```python
from build123d import *

# Parameters (mm, degrees)
SKIZZE1_W                       = 20
SKIZZE1_H                       = 10
AUFSATZ_LINEAR_AUSTRAGEN1_DEPTH = 10
SKIZZE3_W                       = 4.1
SKIZZE3_H                       = 1.9
SCHNITT_LINEAR_AUSTRAGEN2_DEPTH = 5
SKIZZE9_RX                      = 9
SKIZZE9_RY                      = 3
SCHNITT_LINEAR_AUSTRAGEN3_DEPTH = 10
SKIZZE10_W                      = 6.95
SKIZZE10_H                      = 5
SCHNITT_LINEAR_AUSTRAGEN4_DEPTH = 1.5
SKIZZE11_W                      = 7
SKIZZE11_H                      = 5
SCHNITT_LINEAR_AUSTRAGEN5_DEPTH = 1.5
SKIZZE13_W                      = 1
SKIZZE13_H                      = 1
SCHNITT_LINEAR_AUSTRAGEN7_DEPTH = 10
SKIZZE14_W                      = 0.5
SKIZZE14_H                      = 0.5
SCHNITT_LINEAR_AUSTRAGEN8_DEPTH = 10
VERRUNDUNG2_R                   = 0.2
VERRUNDUNG3_R                   = 0.2
VERRUNDUNG4_R                   = 0.2
VERRUNDUNG5_R                   = 0.2
VERRUNDUNG6_R                   = 0.2


with BuildPart() as part:
    # Skizze1 → Aufsatz-Linear austragen1 (new body)
    with BuildSketch(Plane.XY):
        with Locations((-10, 2.346944746)):
            Rectangle(SKIZZE1_W, SKIZZE1_H)
    extrude(amount=AUFSATZ_LINEAR_AUSTRAGEN1_DEPTH)

    # Skizze3 → Schnitt-Linear austragen2 (cut)
    with BuildSketch(Plane(origin=(0, 0, 0), x_dir=(-1, 0, 0), z_dir=(0, 0, -1))):
        with Locations((10, 2.346944746)):
            Rectangle(SKIZZE3_W, SKIZZE3_H)
    extrude(amount=-SCHNITT_LINEAR_AUSTRAGEN2_DEPTH, mode=Mode.SUBTRACT)

    # Skizze9 → Schnitt-Linear austragen3 (cut)
    with BuildSketch(Plane(origin=(0, 7.346944746, 0), x_dir=(1, 0, 0), z_dir=(0, 1, 0))):
        with Locations((-10, -10)):
            Ellipse(SKIZZE9_RX, SKIZZE9_RY)
    extrude(amount=-SCHNITT_LINEAR_AUSTRAGEN3_DEPTH, mode=Mode.SUBTRACT)

    # Skizze10 → Schnitt-Linear austragen4 (cut)
    with BuildSketch(Plane(origin=(0, 0, 0), x_dir=(-1, 0, 0), z_dir=(0, 0, -1))):
        with Locations((16.525, 2.021356222)):
            Rectangle(SKIZZE10_W, SKIZZE10_H)
    extrude(amount=-SCHNITT_LINEAR_AUSTRAGEN4_DEPTH, mode=Mode.SUBTRACT)

    # Skizze11 → Schnitt-Linear austragen5 (cut)
    with BuildSketch(Plane(origin=(0, 0, 0), x_dir=(-1, 0, 0), z_dir=(0, 0, -1))):
        with Locations((3.5, 2.346944746)):
            Rectangle(SKIZZE11_W, SKIZZE11_H)
    extrude(amount=-SCHNITT_LINEAR_AUSTRAGEN5_DEPTH, mode=Mode.SUBTRACT)

    # Skizze13 → Schnitt-Linear austragen7 (cut)
    with BuildSketch(Plane.XZ.offset(2.653055254)):
        with Locations((-10, 6.665824705)):
            Rectangle(SKIZZE13_W, SKIZZE13_H)
    extrude(amount=-SCHNITT_LINEAR_AUSTRAGEN7_DEPTH, mode=Mode.SUBTRACT)

    # Skizze14 → Schnitt-Linear austragen8 (cut)
    with BuildSketch(Plane.XZ.offset(2.653055254)):
        with Locations((-15.25, 7.45)):
            Rectangle(SKIZZE14_W, SKIZZE14_H)
        with Locations((-4.75, 7.45)):
            Rectangle(SKIZZE14_W, SKIZZE14_H)
        with Locations((-13.25, 7.05)):
            Rectangle(SKIZZE14_W, SKIZZE14_H)
        with Locations((-2.75, 8.15)):
            Rectangle(SKIZZE14_W, SKIZZE14_H)
        with Locations((-17.25, 8.15)):
            Rectangle(SKIZZE14_W, SKIZZE14_H)
        with Locations((-6.75, 7.05)):
            Rectangle(SKIZZE14_W, SKIZZE14_H)
    extrude(amount=-SCHNITT_LINEAR_AUSTRAGEN8_DEPTH, mode=Mode.SUBTRACT)

    # Verrundung2
    verrundung2_edges = [part.edges().sort_by_distance(p)[0] for p in [
        (-13.5, 2.346944746, 7.236146008),
        (-15.5, 2.346944746, 7.625365525),
        (-17.5, 2.346944746, 8.341687605),
        (-19, 2.346944746, 10),
    ]]
    fillet(verrundung2_edges, radius=VERRUNDUNG2_R)

    # Verrundung3
    # the kernel refuses this fillet: 0.2 mm, written as the material it takes off along each edge
    with BuildSketch(Plane(origin=(-17, -3.342182333, 8.114381917), x_dir=(0.9302782404562213, 0, -0.3668547332850931), z_dir=(0, 1, 0))) as verrundung3_piece_1:
        with BuildLine():
            CenterArc((0.278646285, 0.199977567), VERRUNDUNG3_R, 180.155482176, 88.986351642)
            Line((0.078647021, 0.199434832), (0.074647036, 0.199423978))
            ThreePointArc((0.074647036, 0.199423978), (0.035602397, 0.101184835), (-0.003721113, 0.001467419))
            Line((-0.003721113, 0.001467419), (6.2365e-05, -0.003999514))
            ThreePointArc((6.2365e-05, -0.003999514), (0.137824964, -0.002947258), (0.275590922, -0.003999551))
            Line((0.275590922, -0.003999551), (0.275650831, 0))
        make_face()
    extrude(amount=11.378254157, mode=Mode.SUBTRACT)
    with BuildSketch(Plane(origin=(-15, -3.272043648, 7.505561742), x_dir=(0.9776339897126725, 0, -0.2103135329893973), z_dir=(0, 1, 0))) as verrundung3_piece_2:
        with BuildLine():
            CenterArc((0.247599452, 0.199994931), VERRUNDUNG3_R, 167.859273294, 101.732777732)
            Line((0.052072654, 0.242057637), (0.048162118, 0.242898891))
            Line((0.048162118, 0.242898891), (-0.003910536, 0.000841254))
            Line((-0.003910536, 0.000841254), (2.8981e-05, -0.003999895))
            ThreePointArc((2.8981e-05, -0.003999895), (0.123087615, -0.00355801), (0.246146974, -0.003999899))
            Line((0.246146974, -0.003999899), (0.246175454, 0))
        make_face()
    extrude(amount=11.237976787, mode=Mode.SUBTRACT)
    with BuildSketch(Plane(origin=(-13, -3.212731809, 7.171572875), x_dir=(0, 0, -1), z_dir=(0, 1, 0))) as verrundung3_piece_3:
        with BuildLine():
            CenterArc((0.223870622, -0.2), VERRUNDUNG3_R, 90, 96.174915405)
            Line((0.025030991, -0.221512819), (0.021054199, -0.221943076))
            ThreePointArc((0.021054199, -0.221943076), (0.008804856, -0.111175678), (-0.003972508, -0.000468165))
            Line((-0.003972508, -0.000468165), (0, 0.004))
            Line((0, 0.004), (0.223870622, 0.004))
            Line((0.223870622, 0.004), (0.223870622, 0))
        make_face()
    extrude(amount=11.119353109, mode=Mode.SUBTRACT)

    # Verrundung4
    # the kernel refuses this fillet: 0.2 mm, written as the material it takes off along each edge
    with BuildSketch(Plane(origin=(-1, 7.805203231, 10), x_dir=(1, 0, 0), z_dir=(0, -1, 0))) as verrundung4_piece_1:
        with BuildLine():
            CenterArc((0.183303394, -0.2), VERRUNDUNG4_R, 90, 80.504337422)
            Line((-0.013956225, -0.167005412), (-0.017901417, -0.16634552))
            ThreePointArc((-0.017901417, -0.16634552), (-0.007497365, -0.083459179), (-0.004, 0))
            Line((-0.004, 0), (0, 0.004))
            Line((0, 0.004), (0.183303394, 0.004))
            Line((0.183303394, 0.004), (0.183303394, 0))
        make_face()
    extrude(amount=10.91651697, mode=Mode.SUBTRACT)
    with BuildSketch(Plane(origin=(-7, -3.212731809, 7.171572875), x_dir=(0, 0, -1), z_dir=(0, 1, 0))) as verrundung4_piece_2:
        with BuildLine():
            CenterArc((0.223870622, 0.2), VERRUNDUNG4_R, 173.825084595, 96.174915405)
            Line((0.025030991, 0.221512819), (0.021054199, 0.221943076))
            ThreePointArc((0.021054199, 0.221943076), (0.008804856, 0.111175678), (-0.003972508, 0.000468165))
            Line((-0.003972508, 0.000468165), (0, -0.004))
            Line((0, -0.004), (0.223870622, -0.004))
            Line((0.223870622, -0.004), (0.223870622, 0))
        make_face()
    extrude(amount=11.119353109, mode=Mode.SUBTRACT)
    with BuildSketch(Plane(origin=(-3, -3.342182333, 8.114381917), x_dir=(0, 0, -1), z_dir=(0, 1, 0))) as verrundung4_piece_3:
        with BuildLine():
            CenterArc((0.288257487, 0.185855858), VERRUNDUNG4_R, 159.336395365, 88.986351642)
            Line((0.101123812, 0.25643197), (0.097381139, 0.257843493))
            ThreePointArc((0.097381139, 0.257843493), (0.04781997, 0.12929678), (-0.003697782, 0.001525257))
            Line((-0.003697782, 0.001525257), (0, -0.004))
            ThreePointArc((0, -0.004), (0.107190958, -0.004), (0.212904405, -0.003717117))
            Line((0.212904405, -0.003717117), (0.214381917, 0))
        make_face()
    extrude(amount=11.378254157, mode=Mode.SUBTRACT)
    with BuildSketch(Plane(origin=(-5, -3.272043648, 7.505561742), x_dir=(0, 0, -1), z_dir=(0, 1, 0))) as verrundung4_piece_4:
        with BuildLine():
            CenterArc((0.247595357, 0.2), VERRUNDUNG4_R, 168.267222268, 101.732777732)
            Line((0.051774029, 0.240669491), (0.047857603, 0.241482881))
            ThreePointArc((0.047857603, 0.241482881), (0.02240856, 0.121082934), (-0.003904338, 0.000869565))
            Line((-0.003904338, 0.000869565), (0, -0.004))
            Line((0, -0.004), (0.247595357, -0.004))
            Line((0.247595357, -0.004), (0.247595357, 0))
        make_face()
    extrude(amount=11.237976787, mode=Mode.SUBTRACT)
    with BuildSketch(Plane(origin=(-6.5, -3.085874245, 7.236146008), x_dir=(0.9896812974841964, 0, 0.1432861801081929), z_dir=(0, 1, 0))) as verrundung4_piece_5:
        with BuildLine():
            CenterArc((0.173129468, 0.19999838), VERRUNDUNG4_R, 188.238048246, 81.531348944)
            Line((-0.024806792, 0.171341144), (-0.028765517, 0.170767999))
            Line((-0.028765517, 0.170767999), (-0.003958725, -0.000573145))
            Line((-0.003958725, -0.000573145), (1.5974e-05, -0.003999968))
            ThreePointArc((1.5974e-05, -0.003999968), (0.086162287, -0.00382729), (0.172308415, -0.003999968))
            Line((0.172308415, -0.003999968), (0.172324514, 0))
        make_face()
    extrude(amount=10.865637981, mode=Mode.SUBTRACT)
    with BuildSketch(Plane(origin=(-4.5, -3.03856184, 7.625365525), x_dir=(0.9671190047653414, 0, 0.2543242627467847), z_dir=(0, 1, 0))) as verrundung4_piece_6:
        with BuildLine():
            CenterArc((0.15420633, 0.199997151), VERRUNDUNG4_R, 194.733548244, 74.960608015)
            Line((-0.039217471, 0.149132298), (-0.043085947, 0.148115001))
            Line((-0.043085947, 0.148115001), (-0.003868476, -0.001017297))
            Line((-0.003868476, -0.001017297), (2.106e-05, -0.003999945))
            ThreePointArc((2.106e-05, -0.003999945), (0.076569439, -0.003797048), (0.153117387, -0.003999943))
            Line((0.153117387, -0.003999943), (0.153138739, 0))
        make_face()
    extrude(amount=10.771013171, mode=Mode.SUBTRACT)
    with BuildSketch(Plane(origin=(-2.5, -2.958042767, 8.341687605), x_dir=(0.8891677006710952, 0, 0.45758146824721596), z_dir=(0, 1, 0))) as verrundung4_piece_7:
        with BuildLine():
            CenterArc((0.122010887, 0.199990312), VERRUNDUNG4_R, 207.231153848, 62.204893345)
            Line((-0.055822654, 0.108474018), (-0.059379324, 0.106643692))
            Line((-0.059379324, 0.106643692), (-0.003556671, -0.001830326))
            Line((-0.003556671, -0.001830326), (3.845e-05, -0.003999815))
            ThreePointArc((3.845e-05, -0.003999815), (0.060021389, -0.003708116), (0.120002981, -0.003999806))
            Line((0.120002981, -0.003999806), (0.120042352, 0))
        make_face()
    extrude(amount=10.609975026, mode=Mode.SUBTRACT)

    # Verrundung5
    verrundung5_edges = [part.edges().sort_by_distance(p)[0] for p in [
        (-9.5, 2.346944746, 7.004633207),
        (-10.5, 2.346944746, 7.004633207),
    ]]
    fillet(verrundung5_edges, radius=VERRUNDUNG5_R)

    # Verrundung6
    verrundung6_edges = [part.edges().sort_by_distance(p)[0] for p in [
        (-20, 2.346944746, 10),
        (0, 2.346944746, 10),
    ]]
    fillet(verrundung6_edges, radius=VERRUNDUNG6_R)


solid = part.part
```
Could you check a few things on this model? Use its own coordinates, in mm. A direction names the side the tool comes from. Give positions to 0.01 mm unless a question says otherwise; leave off trailing zeros. Loops run counter-clockwise (first coordinate to the right, second up) from the corner with the lowest first, then second, coordinate; pieces in that order, holes last. Notation, with made-up numbers: (61, -33.75) - (72, -33.75) arc R20 cw to (72, -12.75) - close; hole circle Ø6 at (47, 16). An arc over 180 degrees is marked (long way). Use one line per item in the form item = value.
1. On a 3-axis mill with a long thin cutter (end or side, diameter ignored), from which of +Z, -Z, +X, -X, +Y, -Y can I reach the whole of each face in a straight line? I mean faces 1 (the face through (-3, 2, 1.5)), 2 (the face through (-7.95, 2, 2)), 3 (the face through (-16, 2, 1.5)). Say none if no direction works.
Response values:
face_1 = -Z, +X
face_2 = -Z
face_3 = -Z, -X
2. I'm going to push flat-ended pins straight in: pin 1 Ø0.6 at (x, y) = (-6.5, 3) entering from +Z; pin 2 Ø2.5 at (x, y) = (-18, 1.5) entering from -Z; pin 3 Ø3 at (x, y) = (-10.5, 3) entering from +Z (3 decimals). Where does each tip first touch, or does it pass through?
Response values:
pin_1 = 7.28
pin_2 = 1.5
pin_3 = 7.075
3. I want a section at C-C (x = -6.75). Please give me the cut outline in (y, z), and give its area (3 significant figures).
Response values:
outline = (-2.65, 0) - (-0.15, 0) - (-0.15, 1.5) - (4.85, 1.5) - (4.85, 0) - (7.35, 0) - (7.35, 6.8) - (-2.65, 6.8) - close
area = 60.5 mm²
4. I want a section at D-D (x = -9.75). Please give me the cut outline in (y, z).
Response values:
outline = (-2.65, 0) - (1.4, 0) - (1.4, 5) - (3.3, 5) - (3.3, 0) - (7.35, 0) - (7.35, 6.17) - (-2.65, 6.17) - close
5. I want a section at B-B (z = 2.25). Please give me the cut outline in (x, y).
Response values:
outline = (-20, -2.65) - (0, -2.65) - (0, 7.35) - (-20, 7.35) - close; hole (-12.05, 1.4) - (-7.95, 1.4) - (-7.95, 3.3) - (-12.05, 3.3) - close
6. I need wall thicknesses on probe 1 along Y at (x, z) = (-11, 3); probe 2 along Y at (x, z) = (-15.25, 0.5); probe 3 along X at (y, z) = (2.25, 1.75). Which ranges of each line are inside material? Lowest first, please.
Response values:
probe_1 = -2.65 to 1.4, 3.3 to 7.35
probe_2 = -2.65 to -0.48, 4.52 to 7.35
probe_3 = -20 to -12.05, -7.95 to 0
7. I want a section at A-A (z = 6.5). Please give me the cut outline in (x, y).
Response values:
outline = (-20, -2.65) - (-10.5, -2.65) - (-10.5, 7.35) - (-20, 7.35) - close; (-9.5, -2.65) - (0, -2.65) - (0, 7.35) - (-9.5, 7.35) - close
8. Thinking about a two-plate mould opening in Y: for faces 4 (the face through (-10, 2, 5)), 5 (the face through (-13.05, 2, 1)), 6 (the face through (-10, 2, 6.166)), 7 (the face through (-10, 7.347, 4)), which applies, released by +Y, released by -Y, zero draft, split by the parting line, or undercut?
Response values:
face_4 = undercut
face_5 = undercut
face_6 = zero draft
face_7 = released by +Y
